Can you work these out from the drawing? Everything is in mm from the part's minimum corner. A direction names the side the tool comes from. Give positions to 0.01 mm unless a question says otherwise; leave off trailing zeros. Order: outer loops, then holes, each group sorted by start corner. A loop starts at its lowest first (then second) coordinate and runs counter-clockwise, first axis right, second up. Notation, with made-up numbers: (45, 60) - (95, 60) arc R29 ccw to (95, 98) - close; hole circle Ø11 at (76.25, 82). An arc over 180 degrees is marked (long way). One line per question, with ' | ' between items.
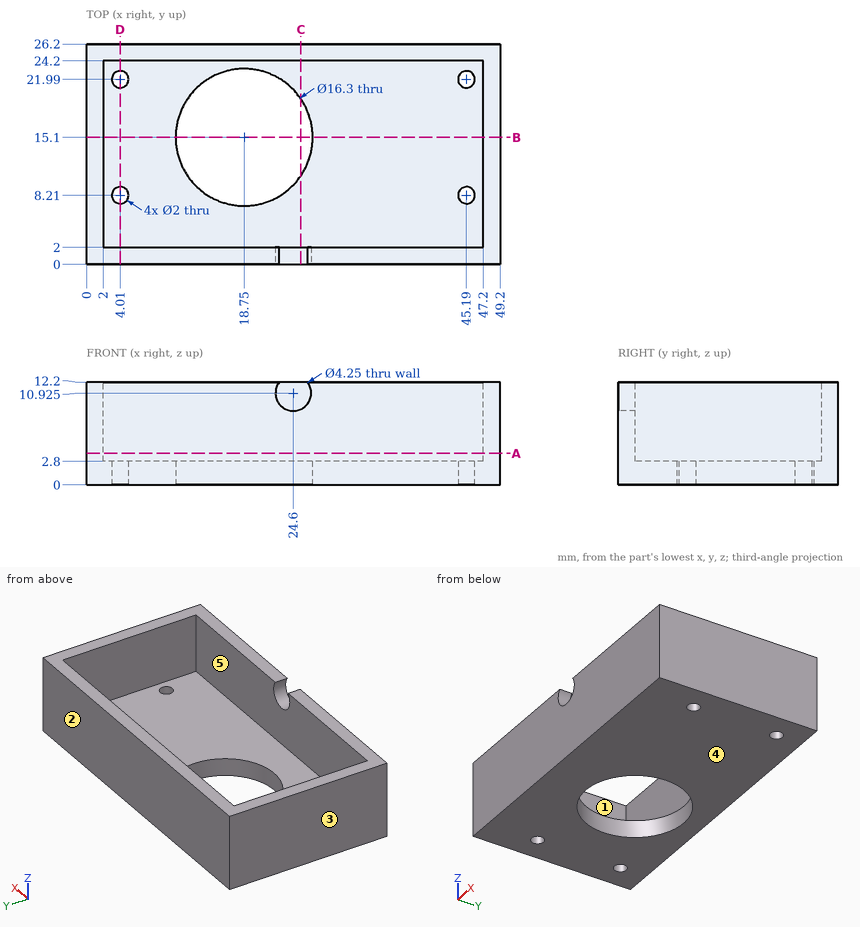
(1) Imagine slicing it at A-A (z = 3.75). List the corners of the cut face in (x, y) for me, and give its area (3 significant figures).
Answer below:
outline: (0, 0) - (49.2, 0) - (49.2, 26.2) - (0, 26.2) - close; hole (2, 2) - (47.2, 2) - (47.2, 24.2) - (2, 24.2) - close | area: 286 mm^2
(2) If we mould it in two halves opening along X, with no side actions, what happens to the marked faces 1, 2 and 3? For each: released by +X, released by -X, zero draft, split by the parting line, or undercut.
Answer below:
face 1: undercut | face 2: zero draft | face 3: released by -X
(3) Imagine slicing it at C-C (x = 25.5). List the corners of the cut face in (y, z) for me.
Answer below:
outline: (0, 0) - (10.53, 0) - (10.53, 2.8) - (2, 2.8) - (2, 9) - (0, 9) - close; (19.67, 0) - (26.2, 0) - (26.2, 12.2) - (24.2, 12.2) - (24.2, 2.8) - (19.67, 2.8) - close
(4) If I drill on line 1 (Y direction, x = 45.19, z = 1.6); line 2 (Y direction, x = 16.5, z = 8); line 3 (X direction, y = 20.5, z = 6.75), over which ranges is the centre line in solid material (lowest first)?
Answer below:
line 1: 0 to 7.21, 9.21 to 20.99, 22.99 to 26.2 | line 2: 0 to 2, 24.2 to 26.2 | line 3: 0 to 2, 47.2 to 49.2
(5) Imagine slicing it at B-B (y = 15.1). List the corners of the cut face in (x, z) for me, and give its area (3 significant figures).
Answer below:
outline: (0, 0) - (10.6, 0) - (10.6, 2.8) - (2, 2.8) - (2, 12.2) - (0, 12.2) - close; (26.9, 0) - (49.2, 0) - (49.2, 12.2) - (47.2, 12.2) - (47.2, 2.8) - (26.9, 2.8) - close | area: 130 mm^2
(6) Will these pins go through, and if not, where does the flat tip stop? pin 1 (1.6 mm diameter, centred on x = 45.19, y = 21.99, fed in from +Z); pin 2 (4 mm diameter, centred on x = 31.5, y = 22, fed in from +Z); pin 3 (12 mm diameter, centred on x = 9.5, y = 18.5, fed in from -Z).
Answer below:
pin 1: through | pin 2: z = 2.8 | pin 3: z = 0
(7) On a 3-axis mill with a long thin cutter (end or side, diameter ignored), from which of +Z, -Z, +X, -X, +Y, -Y can I reach the whole of each face in a straight line? I mean the marked faces 4 and 5. Say none if no direction works.
Answer below:
face 4: -Z, +X, -X, +Y, -Y | face 5: +Z
(8) Imagine slicing it at D-D (x = 4.01). List the corners of the cut face in (y, z) for me.
Answer below:
outline: (0, 0) - (7.21, 0) - (7.21, 2.8) - (2, 2.8) - (2, 12.2) - (0, 12.2) - close; (9.21, 0) - (20.99, 0) - (20.99, 2.8) - (9.21, 2.8) - close; (22.99, 0) - (26.2, 0) - (26.2, 12.2) - (24.2, 12.2) - (24.2, 2.8) - (22.99, 2.8) - close
